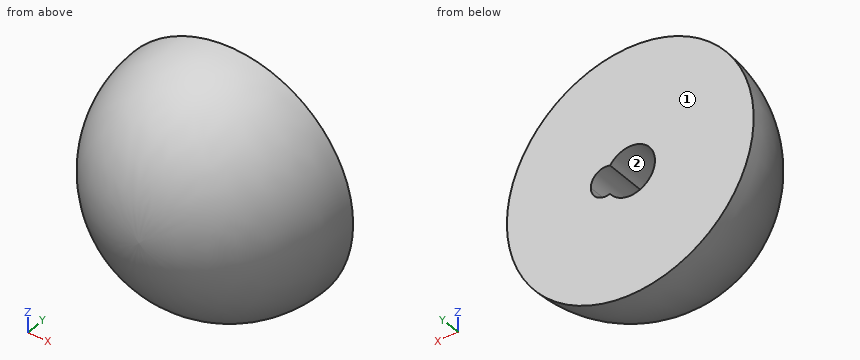
```python
from build123d import *

# Parameters (mm, degrees)
F1_DEPTH = 8
F0_R     = 12.5
F2_R     = 12.5
F3_DEPTH = 12.5
F4_R     = 12.49999
F7_DEPTH = 8


# Not quite as in the source:
# - a fillet or chamfer is up to 0.001 mm smaller than in the source, because OpenCascade refuses the exact size


with BuildPart() as f1:
    # F0 (on Front) → F1 (new body)
    with BuildSketch(Plane.XZ):
        with BuildLine():
            ThreePointArc((0.1338848412, 2.0937357457), (0.1198892217, 2.2981641713), (0.0781635329, 2.4987777937))
            ThreePointArc((0.0781635329, 2.4987777937), (-1.3661151588, 2.0937357457), (-2.3185923934, 0.9349488293))
            ThreePointArc((-2.3185923934, 0.9349488293), (-0.7253015556, 0.7375064414), (0.1338848412, 2.0937357457))
        make_face()
    extrude(amount=F1_DEPTH)


with BuildPart() as f1b:
    # F0 (on Front) → F1, piece 2 (new body)
    with BuildSketch(Plane.XZ):
        Circle(F0_R)
        with BuildLine():
            ThreePointArc((0.0781635329, 2.4987777937), (1.7951892424, 1.7399125219), (2.5, 0))
            ThreePointArc((2.5, 0), (-0.4761927218, -2.4542291033), (-2.3185923934, 0.9349488293))
            ThreePointArc((-2.3185923934, 0.9349488293), (-2.1857842541, 3.3499771931), (0.0781635329, 2.4987777937))
        make_face(mode=Mode.SUBTRACT)
    extrude(amount=F1_DEPTH)


with BuildPart() as f3:
    # F2 (on Front) → F3 (new body)
    with BuildSketch(Plane.XZ):
        Circle(F2_R)
    extrude(amount=F3_DEPTH)

    # F4 (radius 12.5 in the source; OpenCascade refuses exactly that, so slightly less here)
    f4_edges = [f3.edges().sort_by_distance(p)[0] for p in [
        (-12.5, -12.5, 0),
    ]]
    fillet(f4_edges, radius=F4_R)

    # F6 (on Front) → F7 (cut)
    with BuildSketch(Plane.XZ):
        with BuildLine():
            ThreePointArc((2.05, -1.4309088021), (2.3848480035, -0.75), (2.5, 0))
            ThreePointArc((2.5, 0), (2.3848480035, 0.75), (2.05, 1.4309088021))
            ThreePointArc((2.05, 1.4309088021), (1, 0), (2.05, -1.4309088021))
        make_face()
        with BuildLine():
            ThreePointArc((2.05, 1.4309088021), (2.3848480035, 0.75), (2.5, 0))
            ThreePointArc((2.5, 0), (2.3848480035, -0.75), (2.05, -1.4309088021))
            ThreePointArc((2.05, -1.4309088021), (3.3874119675, -1.2093386622), (4, 0))
            ThreePointArc((4, 0), (3.3874119675, 1.2093386622), (2.05, 1.4309088021))
        make_face()
        with BuildLine():
            ThreePointArc((2.05, -1.4309088021), (1, 0), (2.05, 1.4309088021))
            ThreePointArc((2.05, 1.4309088021), (-2.5, 0), (2.05, -1.4309088021))
        make_face()
    extrude(amount=F7_DEPTH, mode=Mode.SUBTRACT)


solid = f3.part
```
Check sheet for the modelled part. Datum: model origin and axes. Units: mm. Face numbers are marked on the shaded views. Round coordinates to 2 decimals unless told otherwise and drop trailing zeros. Answer in a Markdown table with one row per item.
Q1. Go/stop test with flat-tipped pins: P1, Ø4, axis at y = -3, z = -6.5, coming from the +X side; P2, Ø12, axis at x = -7, z = -6, coming from the -Y side; P3, Ø4, axis at x = -1.5, z = -8.5, coming from the -Y side. Record where each tip stops, or that it passes through.
Data:
| item | result |
|---|---|
| P1 | stops at x = 11.39 |
| P2 | stops at y = -12.08 |
| P3 | stops at y = -10.6 |
Q2. Thickness scan on L1, parallel to Z at x = 0, y = -2; L2, parallel to Z at x = 0, y = -5.5. Record the ranges inside material, lowest first.
Data:
| item | result |
|---|---|
| L1 | z = -12.34 to -2.5, 2.5 to 12.34 |
| L2 | z = -11.22 to -2.5, 2.5 to 11.22 |
Q3. Release check for a two-part mould opening along Z. For the marked faces 1 and 2 record: released by +Z, released by -Z, zero draft, split by the parting line, or undercut.
Data:
| item | result |
|---|---|
| face 1 | zero draft |
| face 2 | undercut |
